Autodesk Inventor part; units mm, degrees
ref_plane "Work Plane1" through (-1.5, 1, -12.5) normal (-1, 0, 0) x (0, 0, 1)
ref_plane "YZ Plane" through (0, 0, 0) normal (1, 0, 0) x (0, 1, 0)
ref_plane "XZ Plane" through (0, 0, 0) normal (0, 1, 0) x (-1, 0, 0)
sketch "Sketch1" plane through (0, 0, 0) normal (0, 0, 1) x (1, 0, 0)
  line L0 (-6, 1) -> (6, 1)
  line L1 (6, 1) -> (6, -1)
  line L2 (6, -1) -> (-6, -1)
  line L3 (-6, -1) -> (-6, 1)
  line L4 (-6, 1) -> (6, -1) construction
  line L5 (6, 1) -> (-6, -1) construction
  line L6 (-6, -1) -> (-6, -3)
  line L7 (6, -1) -> (6, -3)
  arc A0 (6, -3) -> (-6, -3) centre (0, -11) ccw
  point P0 (0, 0)
  dimension "d0" = 12
  dimension "d1" = 2
  dimension "d2" = 2
  dimension "d3" = 2
extrude "Extrusion1" add sketch "Sketch1" against normal blind 25
sketch "Sketch2" plane through (-6, 1, 0) normal (0, 1, 0) x (1, 0, 0)
  line L0 (12, 0) -> (12, 25)
  line L1 (0, 0) -> (0, 25)
  line L2 (0, 0) -> (0, 2.5)
  line L3 (12, 0) -> (12, 2.5)
  line L4 (0, 25) -> (0, 22.5)
  line L5 (12, 25) -> (12, 22.5)
  line L6 (0, 2.5) -> (4.5, 2.5)
  line L7 (4.5, 2.5) -> (4.5, 22.5)
  line L8 (4.5, 22.5) -> (0, 22.5)
  line L9 (0, 22.5) -> (0, 2.5)
  line L10 (12, 2.5) -> (7.5, 2.5)
  line L11 (7.5, 2.5) -> (7.5, 22.5)
  line L12 (7.5, 22.5) -> (12, 22.5)
  line L13 (12, 22.5) -> (12, 2.5)
  point P0 (6, 0)
  dimension "d6" = 2.5
  dimension "d7" = 2.5
  dimension "d8" = 2.5
  dimension "d9" = 2.5
  dimension "d10" = 12
  dimension "d11" = 4.5
  dimension "d12" = 4.5
extrude "Extrusion2" cut sketch "Sketch2" against normal blind 25
sketch "Sketch3" plane through (-6, 1, 0) normal (0, 1, 0) x (1, 0, 0)
  line L0 (7.5, 2.5) -> (7.5, 22.5)
  line L1 (4.5, 22.5) -> (4.5, 2.5)
  line L2 (0, 0) -> (0, 2.5)
  line L3 (4.5, 2.5) -> (4.5, 3.5)
  line L4 (7.5, 2.5) -> (7.5, 3.5)
  line L5 (4.5, 3.5) -> (4.5, 5)
  line L6 (4.5, 5) -> (5, 5)
  line L7 (5, 5) -> (5, 3.5)
  line L8 (5, 3.5) -> (4.5, 3.5)
  line L9 (7.5, 3.5) -> (7.5, 5)
  line L10 (7.5, 5) -> (7, 5)
  line L11 (7, 5) -> (7, 3.5)
  line L12 (7, 3.5) -> (7.5, 3.5)
  line L13 (4.5, 2.5) -> (4.5, 7)
  line L14 (4.5, 7) -> (0, 7)
  line L15 (0, 7) -> (0, 8.5)
  line L16 (0, 8.5) -> (4.5, 8.5)
  line L17 (7.5, 7) -> (12, 7)
  line L18 (12, 7) -> (12, 8.5)
  line L19 (12, 8.5) -> (7.5, 8.5)
  line L20 (4.5, 7) -> (4.5, 21)
  line L21 (7.5, 7) -> (7.5, 21)
  line L22 (4.5, 21) -> (7.5, 21)
  line L23 (7.5, 21) -> (7.5, 22.5)
  line L24 (7.5, 22.5) -> (4.5, 22.5)
  line L25 (4.5, 22.5) -> (4.5, 21)
  line L26 (4.5, 21) -> (3.5, 21)
  line L27 (3.5, 21) -> (3.5, 11)
  line L28 (3.5, 11) -> (4.5, 11)
  line L29 (4.5, 11) -> (4.5, 21)
  line L30 (7.5, 21) -> (8.5, 21)
  line L31 (8.5, 21) -> (8.5, 11)
  line L32 (8.5, 11) -> (7.5, 11)
  line L33 (7.5, 11) -> (7.5, 21)
  line L34 (3.5, 21) -> (4.5, 22.5)
  line L35 (7.5, 22.5) -> (8.5, 21)
  line L36 (7.5, 5) -> (8, 5)
  line L37 (8, 5) -> (8, 3.5)
  line L38 (8, 3.5) -> (7.5, 3.5)
  line L39 (4.5, 5) -> (4, 5)
  line L40 (4, 5) -> (4, 3.5)
  line L41 (4, 3.5) -> (5, 3.5)
  point P0 (12, 25)
  point P1 (12, 0)
  point P2 (6, 0)
  dimension "d15" = 1
  dimension "d16" = 1.5
  dimension "d17" = 0.5
  dimension "d18" = 0.5
  dimension "d19" = 4.5
  dimension "d20" = 1.5
  dimension "d21" = 14
  dimension "d22" = 4.5
  dimension "d23" = 4.5
  dimension "d24" = 14
  dimension "d25" = 25
  dimension "d26" = 1.5
  dimension "d29" = 1
  dimension "d30" = 10
  dimension "d31" = 1
  dimension "d34" = 0.5
  dimension "d35" = 0.5
  dimension "d50" = 10
extrude "Extrusion3" add sketch "Sketch3" along normal blind 4 contours L0 L30 L31 L32 | L22 L1 L24 L0 | L0 L35 L30 | L26 L34 L1 | L1 L28 L27 L26
ref_plane "Work Plane1" through (-1.5, 1, -12.5) normal (-1, 0, 0) x (0, 0, 1)
sketch "Sketch8" plane through (-2.5, -1.3175, -11) normal (-1, 0, 0) x (0, 0, 1)
  line L0 (-10, 6.3175) -> (-11.5, 6.3175)
  line L1 (0, 0) -> (-10, 0)
  line L2 (0, 2.3175) -> (0, 6.3175)
  line L3 (-10, 6.3175) -> (0, 6.3175)
  line L4 (-10, 2.3175) -> (0, 2.3175)
  line L5 (-3, 6.3175) -> (-1, 6.3175)
  line L6 (-3, 2.3175) -> (-1, 2.3175)
  line L7 (0, 2.3175) -> (-10, 2.3175)
  line L8 (0, 2.3175) -> (-10, 2.3175)
  line L9 (-3, 6.3175) -> (-3, 2.3175)
  line L10 (-1, 2.3175) -> (-1, 6.3175)
  point P0 (11, 1.3175)
  dimension "d119" = 4
  dimension "d120" = 4
  dimension "d126" = 1
  dimension "d127" = 2
sketch "Sketch9" plane through (2.5, -1.3175, -21) normal (1, 0, 0) x (0, 0, -1)
  line L0 (0, 2.3175) -> (0, 6.3175)
  line L1 (0, 0) -> (-10, 0)
  line L2 (-10, 2.3175) -> (0, 2.3175)
  line L3 (-9, 2.3175) -> (-9, 6.3175)
  line L4 (-9, 5.1588) -> (-9, 6.3175)
  line L5 (-9, 6.3175) -> (-7, 6.3175)
  line L6 (-10, 6.3175) -> (0, 6.3175)
  line L7 (-9, 6.3175) -> (-9, 2.3175)
  line L8 (-9, 2.3175) -> (-7, 2.3175)
  line L9 (-10, 6.3175) -> (0, 6.3175)
  line L10 (0, 6.3175) -> (-10, 6.3175)
  line L11 (-10, 6.3175) -> (-9, 6.3175)
  line L12 (-7, 2.3175) -> (-7, 6.3175)
  line L13 (-7, 6.3175) -> (-7, 2.3175)
  point P0 (-21, 1.3175)
  point P1 (-9, 1.1588)
  dimension "d121" = 4
  dimension "d122" = 1
  dimension "d123" = 2
ref_plane "Work Plane2" through (-1.5, 5, -11) normal (-1, 0, 0) x (0, 0, -1)
sketch "Sketch12" plane through (-1.5, 5, -11) normal (-1, 0, 0) x (0, 0, -1)
  line L0 (11.5, 4) -> (11.5, 0)
  line L1 (14, 8) -> (14, 4)
  line L2 (14, 4) -> (11.5, 0)
  line L3 (11.5, 4) -> (14, 4)
  line L4 (14, 0) -> (11.5, 0)
  line L5 (11.5, 0) -> (13.6217, 0) construction
  line L6 (13.6217, 0) -> (14.1176, 2) construction
  line L7 (14.1176, 2) -> (14, 4) construction
  spline S0 degree 3 poles (11.5, 0) (13.6217, 0) (14.1176, 2) (14, 4) knots 1 1 1 1 2 2 2 2
  point P0 (-11, 5)
extrude "Extrusion12" add sketch "Sketch12" against normal up to surface (3 mm away)
sketch "Sketch15" plane through (2.5, -1.3175, -21) normal (1, 0, 0) x (0, 0, -1)
  line L0 (1.5, 2.3175) -> (4, 2.3175)
  line L1 (1.5, 2.3175) -> (1.5, 6.3175)
  line L2 (4, 2.3175) -> (1.5, 2.3175)
  line L3 (1.5, 2.3175) -> (1.5, 3.3175)
  circle A0 centre (1.5, 3.3175) radius 1.3
  point P0 (-21, 1.3175)
  dimension "d77" = 1
  dimension "d78" = 2.6
extrude "Extrusion14" cut sketch "Sketch15" against normal up to surface (12 mm away) from surface at 3.5
sketch "Sketch16" plane through (-6, 5, 0) normal (0, 1, 0) x (1, 0, 0)
  line L0 (3.5, 11) -> (4.5, 11)
  line L1 (4.5, 11) -> (4.5, 21)
  line L2 (7.5, 21) -> (7.5, 11)
  line L3 (7.5, 11) -> (8.5, 11)
  line L4 (4.5, 11) -> (4.3, 11)
  line L5 (4.3, 11) -> (4.3, 21)
  line L6 (4.3, 21) -> (4.5, 21)
  line L7 (7.5, 11) -> (7.5, 21)
  line L8 (7.5, 11) -> (7.7, 11)
  line L9 (7.7, 11) -> (7.7, 21)
  line L10 (7.7, 21) -> (7.5, 21)
  line L11 (7.5, 21) -> (7.5, 11)
  point P0 (6, 0)
  dimension "d81" = 0.2
  dimension "d82" = 0.2
  dimension "d83" = 0.2
extrude "Extrusion15" cut sketch "Sketch16" against normal up to surface (4 mm away)
sketch "Sketch20" plane through (6, -3, 0) normal (1, 0, 0) x (0, 0, -1)
  line L0 (0, 4) -> (2.5, 4)
  line L1 (0, 4) -> (4.5, 4)
  arc A0 (4.5, 5) -> (0, 5) centre (2.25, 5) ccw
  line L2 (4.5, 4) -> (4.5, 5)
  line L3 (0, 4) -> (0, 5)
  line L4 (0, 4) -> (0, 5)
  arc A1 (4.5, 5) -> (0, 5) centre (2.25, 5) ccw
  line L5 (22.5, 1.8869) -> (2.5, 1.8869)
  line L6 (2.5, 1.8869) -> (4.5, 4)
  line L7 (2.5, 1.8869) -> (22.5, 1.8869)
  line L8 (21, 4) -> (2.5, 4)
  line L9 (2.5, 1.8869) -> (2.5, 4)
  point P0 (0, 3)
extrude "Extrusion18" add sketch "Sketch20" against normal blind 2.5
sketch "Sketch21" plane through (-6, -3, 0) normal (-1, 0, 0) x (0, 0, 1)
  arc A0 (0, 5) -> (-4.5, 5) centre (-2.25, 5) ccw
  line L0 (-4.5, 5) -> (-4.5, 4)
  line L1 (-21, 4) -> (-2.5, 4)
  line L2 (0, 4) -> (0, 5)
  line L3 (0, 4) -> (-4.5, 4)
  line L4 (-4.5, 5) -> (-4.5, 4)
  line L5 (0, 0) -> (0, 5)
  line L6 (0, 4) -> (0, 5)
  arc A1 (0, 5) -> (-4.5, 5) centre (-2.25, 5) ccw
  line L7 (-2.5, 4) -> (-2.5, 0)
  line L8 (-2.5, 1.8869) -> (-22.5, 1.8869)
  line L9 (-4.5, 4) -> (-2.5, 1.8869)
  line L10 (-4.5, 4) -> (-2.5, 1.8869)
  line L11 (-2.5, 1.8869) -> (-2.5, 4)
  point P0 (0, 3)
extrude "Extrusion19" add sketch "Sketch21" against normal blind 2.5
sketch "Sketch22" plane through (6, -3, 0) normal (1, 0, 0) x (0, 0, -1)
  arc A0 (4.5, 5) -> (0, 5) centre (2.25, 5) ccw
  circle A1 centre (2.25, 5) radius 1.5
  point P0 (0, 3)
  dimension "d111" = 3
extrude "Extrusion20" cut sketch "Sketch22" against normal up to surface (2.5 mm away)
sketch "Sketch23" plane through (-6, -3, -2.5) normal (-1, 0, 0) x (0, 0, 1)
  arc A0 (2.5, 5) -> (-2, 5) centre (0.25, 5) ccw
  circle A1 centre (0.25, 5) radius 1.5
  point P0 (2.5, 3)
  dimension "d114" = 3
extrude "Extrusion21" cut sketch "Sketch23" against normal up to surface (2.5 mm away)
sketch "Sketch24" plane through (-6, 1, 0) normal (0, -1, 0) x (1, 0, 0)
  line L0 (4.3, -21) -> (4.3, -11)
  line L1 (3.5, -11) -> (4.3, -11)
  line L2 (3.5, -21) -> (3.5, -11)
  line L3 (3.9462, -21.6693) -> (3.5, -21)
  line L4 (3.9462, -21.6693) -> (4.5, -21.6693)
  line L5 (4.5, -21.6693) -> (4.5, -21)
  line L6 (4.5, -21) -> (4.3, -21)
  line L7 (7.5, -22.5) -> (7.5, -2.5)
  line L8 (7.7, -21) -> (7.5, -21)
  line L9 (7.5, -21) -> (7.5, -21.6693)
  line L10 (7.5, -21.6693) -> (8.0538, -21.6693)
  line L11 (8.5, -21) -> (8.0538, -21.6693)
  line L12 (8.5, -11) -> (8.5, -21)
  line L13 (7.7, -11) -> (8.5, -11)
  line L14 (7.7, -11) -> (7.7, -21)
  line L15 (0, -23.3307) -> (4.5, -23.3307)
  line L16 (0, -22.5) -> (0, -23.3307)
  line L17 (4.5, -22.5) -> (0, -22.5)
  line L18 (4.5, -21.6693) -> (4.5, -22.5)
  line L19 (3.9462, -21.6693) -> (4.5, -21.6693)
  line L20 (4.5, -22.5) -> (3.9462, -21.6693)
  line L21 (4.5, -23.3307) -> (4.5, -22.5)
  line L22 (7.5, -23.3307) -> (12, -23.3307)
  line L23 (7.5, -22.5) -> (7.5, -23.3307)
  line L24 (8.0538, -21.6693) -> (7.5, -22.5)
  line L25 (7.5, -21.6693) -> (8.0538, -21.6693)
  line L26 (7.5, -22.5) -> (7.5, -21.6693)
  line L27 (12, -22.5) -> (7.5, -22.5)
  line L28 (12, -23.3307) -> (12, -22.5)
  line L29 (7.5, -2.5) -> (12, -2.5)
  line L30 (12, 0) -> (12, -2.5)
  line L31 (0, 0) -> (12, 0)
  line L32 (0, 0) -> (0, -2.5)
  line L33 (0, -2.5) -> (4.5, -2.5)
  line L34 (4.5, -2.5) -> (4.5, -22.5)
  line L35 (4.5, -22.5) -> (0, -22.5)
  line L36 (0, -22.5) -> (0, -25)
  line L37 (12, -25) -> (0, -25)
  line L38 (12, -22.5) -> (12, -25)
  line L39 (12, -22.5) -> (7.5, -22.5)
  line L40 (7.5, -22.5) -> (7.5, -2.5)
  line L41 (7.5, -2.5) -> (12, -2.5)
  line L42 (12, 0) -> (12, -2.5)
  line L43 (0, 0) -> (12, 0)
  line L44 (0, 0) -> (0, -2.5)
  line L45 (0, -2.5) -> (4.5, -2.5)
  line L46 (4.5, -2.5) -> (4.5, -22.5)
  line L47 (4.5, -22.5) -> (0, -22.5)
  line L48 (0, -22.5) -> (0, -25)
  line L49 (12, -25) -> (0, -25)
  line L50 (12, -22.5) -> (12, -25)
  line L51 (12, -22.5) -> (7.5, -22.5)
  line L52 (7.5, -22.5) -> (7.5, -2.5)
  line L53 (4.5, -30) -> (4.5, 5)
  line L54 (8.5, -11) -> (7.5, -11)
  line L55 (7.5, -2.5) -> (7.5, -21)
  line L56 (7.5, -22.5) -> (4.5, -22.5)
  line L57 (7.5, -11) -> (7.5, -22.5)
  line L58 (8.3667, -21.2) -> (7.5, -22.5)
  line L59 (7.5, -22.5) -> (8.5, -21)
  line L60 (8.5, -11) -> (8.5, -21)
  line L61 (8.5, -11) -> (8.5, -21)
  line L62 (8.5, -11) -> (8.5, -21)
  line L63 (7.5, -11) -> (7.5, -22.5)
  line L64 (3.5, -21) -> (3.5, -11)
  line L65 (3.5, -11) -> (3.5, -21)
  line L66 (3.5, -21) -> (3.5, -11)
  line L67 (3.5, -21) -> (4.5, -22.5)
  line L68 (3.5, -11) -> (4.5, -11)
  line L69 (3.5, -21) -> (4.5, -22.5)
  line L70 (4.5, -22.5) -> (4.5, -11)
  line L71 (4.5, -2.5) -> (4.5, -22.5)
  line L72 (4.5, -11) -> (4.5, -22.5)
  point P0 (6, 0)
  point P1 (3.5, -12)
  point P2 (3.5, -14)
  point P3 (8.5, -14)
  point P4 (8.5, -12)
extrude "Extrusion22" add sketch "Sketch24" along normal blind 1 contours L6 L5 L4 L3 L2 L1 L0 | L0 L68 L34 L6 | L18 L20 L4 | L7 L10 L24 | L7 L8 L14 L13 L12 L11 L10 | L7 L54 L14 L8
extrude "Extrusion23" add sketch "Sketch9" along normal blind 3 contours L2 L3 L5 L12
extrude "Extrusion24" add sketch "Sketch8" along normal blind 3 contours L4 L9 L3 L10
equation "\"d7\" = d6"
equation "\"d8\" = d6"
equation "\"d9\" = d6"
equation "\"d12\" = d11"
equation "\"d18\" = d17"
equation "\"d22\" = d23"
equation "\"d24\" = d21"
equation "\"d31\" = d29"
equation "\"d34\" = d17"
equation "\"d50\" = d30"
equation "\"d82\" = d81"
properties part number "back_pack_5"
CAD build for the part. Positions are in the model's coordinates, mm. A direction names the side the tool comes from. Give positions to 0.01 mm unless a question says otherwise; leave off trailing zeros. Order: outer loops, then holes, each group sorted by start corner. A loop starts at its lowest first (then second) coordinate and runs counter-clockwise, first axis right, second up.
(1) Tool access for faces 5 (the flat face through (-3, -1, -2.5)), 6 (the flat face through (-4, 1, -13)), 7 (the flat face through (1.7, 3, -16)), 8 (the flat face through (4, 3, -14)): list every direction of +Z, -Z, +X, -X, +Y, -Y with a clear straight run to the whole face (end or side of a thin tool).
(2) Saw through at A-A, the plane z = -3.5. Give the cut face in (x, y).
(3) Saw through at D-D, the plane z = -19. Give the cut face in (x, y), then the cut area to 3 significant figures.
(4) Saw through at C-C, the plane x = -2.75. Give the cut face in (y, z).
(5) Flat gauge pins, fed straight in: pin 1 (3 mm diameter, centred on y = -1.5, z = -7, fed in from +X); pin 2 (1.2 mm diameter, centred on x = -3.5, y = -0.5, fed in from -Z); pin 3 (2.5 mm diameter, centred on y = 1.5, z = -15.5, fed in from -X); pin 4 (3 mm diameter, centred on y = 2, z = -23.5, fed in from +X). Where does each tip first touch, or does it go through?
(6) Saw through at B-B, the plane y = -2. Give the cut face in (x, z), then the cut area to 3 significant figures.
(7) Mould opens along Z. For faces 1 (the flat face through (-2, 0, -17)), 2 (the flat face through (-0.1, -0.5, -25)), 3 (the flat face through (-6, 0, -2)), 4 (the flat face through (-4, 3, -12)) say: released by +Z, released by -Z, zero draft, split by the parting line, or undercut.
(8) Drill centre lines: L1, parallel to Z at x = -4.4, y = 2; L2, parallel to X at y = 4, z = -16.25; L3, parallel to X at y = -0.75, z = -14.75. Where is each one in solid material? Low to high.
Results found:
1. face 5: -Y
1. face 6: -X, -Y
1. face 7: +Z, +Y
1. face 8: -Z, +X, +Y, -Y
2. outline: (-6, -0.06) - (-3.5, -0.06) - (-3.5, 1.17) - (-6, 1.17) - close; (-6, 2.83) - (-3.5, 2.83) - (-3.5, 3.87) - (-6, 3.87) - close; (-1.5, -1.11) arc R10 cw to (1.5, -1.11) - (1.5, 1) - (-1.5, 1) - close; (3.5, -0.06) - (6, -0.06) - (6, 1.17) - (3.5, 1.17) - close; (3.5, 2.83) - (6, 2.83) - (6, 3.87) - (3.5, 3.87) - close
3. outline: (-2.5, 0) - (-1.5, 0) - (-1.5, -1.11) arc R10 cw to (1.5, -1.11) - (1.5, 0) - (2.5, 0) - (2.5, 5) - (1.7, 5) - (1.7, 1) - (-1.7, 1) - (-1.7, 5) - (-2.5, 5) - close
3. area: 14.5 mm2
4. outline: (-1.39, -25) - (1, -25) - (1, -23.33) arc R1.3 cw to (0.7, -22.5) - (-1.39, -22.5) - close; (-1.39, -2.5) - (1, -2.5) - (1, 0) - (-1.39, 0) - close; (1, -14) - (5, -14) - (5, -12) - (1, -12) - close
5. pin 1: stops at x = 1.5
5. pin 2: stops at z = -25
5. pin 3: stops at x = -2.5
5. pin 4: stops at x = 6
6. outline: (-6, -25) - (-4.36, -25) - (-4.36, -22.5) - (-6, -22.5) - close; (-6, -2.5) - (-4.36, -2.5) - (-4.36, 0) - (-6, 0) - close; (4.36, -25) - (6, -25) - (6, -22.5) - (4.36, -22.5) - close; (4.36, -2.5) - (6, -2.5) - (6, 0) - (4.36, 0) - close
6. area: 16.4 mm2
7. face 1: undercut
7. face 2: released by -Z
7. face 3: zero draft
7. face 4: undercut
8. L1: z = -14 to -12, -4.5 to -3.75, -0.75 to 0
8. L2: x = -2.5 to -1.7, 1.7 to 2.5
8. L3: x = -1.5 to 1.5
